Input: dimensioned drawing with shaded views. Units: mm. Origin: part minimum x, y, z. Give positions to 0.01 mm unless a question says otherwise; leave off trailing zeros. Order: outer loops, then holes, each group sorted by start corner. A loop starts at its lowest first (then second) coordinate and runs counter-clockwise, first axis right, second up. Notation, with made-up numbers: (43.25, 82.25) -> (85.25, 82.25) arc R10 ccw to (85.25, 92.25) -> close; hole circle Ø6 at (57, -3.5). An arc over 180 degrees is marked (long way). One line per question, with ' | ' between items. Start each with the question number.
(1) Section A-A (y = 17.25). Return loops of the section in (x, z).
(2) Section B-B (x = 67.5). Return loops of the section in (y, z).
(3) Ray query, L1, parallel to X at y = 0.9, z = 46.5; L2, parallel to Z at x = 2.5, y = 1.4; L3, parallel to Z at x = 4, y = 1.5. Return the intervals inside material, ascending.
(4) Section C-C (z = 25). Return loops of the section in (x, y), then the cut area to 3 significant figures.
(5) First-contact query: pin 1 Ø6 at (x, y) = (74.5, 17) entering from +Z; pin 2 Ø5 at (x, z) = (27, 12) entering from +Y; pin 3 Ø6 at (y, z) = (18.5, 23.5) entering from -X; pin 4 Ø5 at (x, y) = (60.5, 7.5) entering from -Z. Flat tips, straight axial feed; report the tip coordinate or a pass-through.
(6) Section D-D (x = 76). Return loops of the section in (y, z), then the cut area to 3 significant figures.
(7) Mould query, pull axis Z, two halves, no side actions, for the marked faces 1, 2 and 3. Classes: +Z half, -Z half, draft (parallel to the pull), parting line (faces both ways), or undercut.
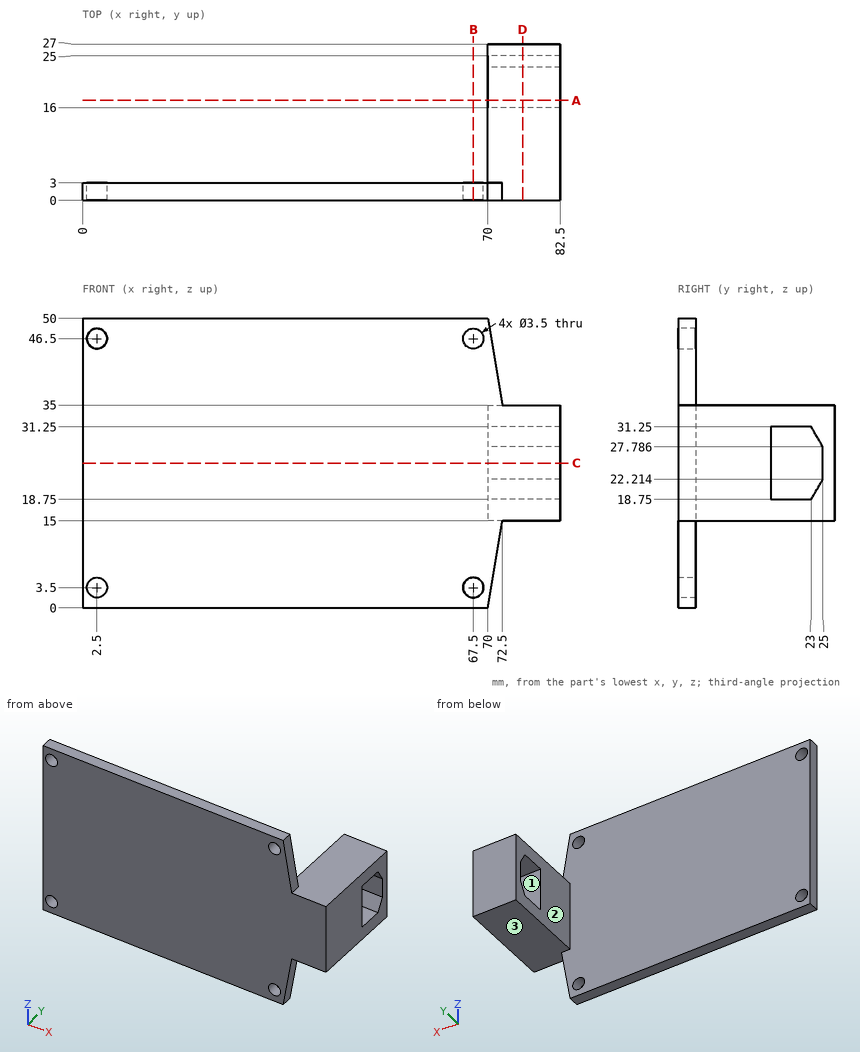
Response:
1) outline: (70, 15) -> (82.5, 15) -> (82.5, 18.75) -> (70, 18.75) -> close; (70, 31.25) -> (82.5, 31.25) -> (82.5, 35) -> (70, 35) -> close
2) outline: (0, 0) -> (3, 0) -> (3, 1.75) -> (0, 1.75) -> close; (0, 5.25) -> (3, 5.25) -> (3, 44.75) -> (0, 44.75) -> close; (0, 48.25) -> (3, 48.25) -> (3, 50) -> (0, 50) -> close
3) L1: x = 0 to 0.75, 4.25 to 65.75, 69.25 to 70.58 | L2: z = 0 to 1.75, 5.25 to 44.75, 48.25 to 50 | L3: z = 0 to 2.6, 4.4 to 45.6, 47.4 to 50
4) outline: (0, 0) -> (82.5, 0) -> (82.5, 16) -> (70, 16) -> (70, 3) -> (0, 3) -> close; (70, 25) -> (82.5, 25) -> (82.5, 27) -> (70, 27) -> close | area: 435 mm^2
5) pin 1: stops at z = 35 | pin 2: stops at y = 3 | pin 3: stops at x = 70 | pin 4: passes through
6) outline: (0, 15) -> (27, 15) -> (27, 35) -> (0, 35) -> close; hole (16, 18.75) -> (23, 18.75) -> (25, 22.21) -> (25, 27.79) -> (23, 31.25) -> (16, 31.25) -> close | area: 434 mm^2
7) face 1: undercut | face 2: draft | face 3: -Z half
